Geometry check sheet. Reference: the model listing, model coordinates, mm. A direction names the side the tool comes from. Coordinates: 2 decimals unless noted, no trailing zeros. Loops run counter-clockwise (first coordinate to the right, second up) from the corner with the lowest first, then second, coordinate; pieces in that order, holes last. Notation, with made-up numbers: (13.25, -20.75) -> (35.25, -20.75) arc R24 ccw to (35.25, 8.25) -> close; hole circle Ø1 at (-14.5, 89). An arc over 180 degrees is marked (long way). Answer as a JSON object with one key per item and string values.
from build123d import *

# Parameters (mm, degrees)
F0_R     = 48.035646
F1_DEPTH = 18


with BuildPart() as f1:
    # F0 (on Front) → F1 (new body)
    with BuildSketch(Plane.XZ):
        Polygon((-1152.091861, -39.495662), (52.929014, -39.495662), (52.929014, 361.01982), (-1152.091861, 1360.379338), align=None)
        with Locations((-1022.033925, 72.34408)):
            Circle(F0_R, mode=Mode.SUBTRACT)
        with Locations((-862.033925, 72.34408)):
            Circle(F0_R, mode=Mode.SUBTRACT)
        with Locations((-1022.033925, 232.34408)):
            Circle(F0_R, mode=Mode.SUBTRACT)
        with Locations((-862.033925, 232.34408)):
            Circle(F0_R, mode=Mode.SUBTRACT)
        with Locations((-702.033925, 72.34408)):
            Circle(F0_R, mode=Mode.SUBTRACT)
        with Locations((-702.033925, 232.34408)):
            Circle(F0_R, mode=Mode.SUBTRACT)
        with Locations((-1022.033925, 392.34408)):
            Circle(F0_R, mode=Mode.SUBTRACT)
        with Locations((-862.033925, 392.34408)):
            Circle(F0_R, mode=Mode.SUBTRACT)
        with Locations((-1022.033925, 552.34408)):
            Circle(F0_R, mode=Mode.SUBTRACT)
        with Locations((-862.033925, 552.34408)):
            Circle(F0_R, mode=Mode.SUBTRACT)
        with Locations((-702.033925, 392.34408)):
            Circle(F0_R, mode=Mode.SUBTRACT)
        with Locations((-702.033925, 552.34408)):
            Circle(F0_R, mode=Mode.SUBTRACT)
        with Locations((-542.033925, 72.34408)):
            Circle(F0_R, mode=Mode.SUBTRACT)
        with Locations((-382.033925, 72.34408)):
            Circle(F0_R, mode=Mode.SUBTRACT)
        with Locations((-542.033925, 232.34408)):
            Circle(F0_R, mode=Mode.SUBTRACT)
        with Locations((-382.033925, 232.34408)):
            Circle(F0_R, mode=Mode.SUBTRACT)
        with Locations((-222.033925, 72.34408)):
            Circle(F0_R, mode=Mode.SUBTRACT)
        with Locations((-62.033925, 72.34408)):
            Circle(F0_R, mode=Mode.SUBTRACT)
        with Locations((-222.033925, 232.34408)):
            Circle(F0_R, mode=Mode.SUBTRACT)
        with Locations((-62.033925, 232.34408)):
            Circle(F0_R, mode=Mode.SUBTRACT)
        with Locations((-542.033925, 392.34408)):
            Circle(F0_R, mode=Mode.SUBTRACT)
        with Locations((-382.033925, 392.34408)):
            Circle(F0_R, mode=Mode.SUBTRACT)
        with Locations((-542.033925, 552.34408)):
            Circle(F0_R, mode=Mode.SUBTRACT)
        with Locations((-382.033925, 552.34408)):
            Circle(F0_R, mode=Mode.SUBTRACT)
        with Locations((-222.033925, 392.34408)):
            Circle(F0_R, mode=Mode.SUBTRACT)
        with Locations((-1022.033925, 712.34408)):
            Circle(F0_R, mode=Mode.SUBTRACT)
        with Locations((-862.033925, 712.34408)):
            Circle(F0_R, mode=Mode.SUBTRACT)
        with Locations((-702.033925, 712.34408)):
            Circle(F0_R, mode=Mode.SUBTRACT)
        Polygon((-588.994136, 827.545822), (-1101.989508, 827.545822), (-1101.989508, 1252.988085), align=None, mode=Mode.SUBTRACT)
        with Locations((-542.033925, 712.34408)):
            Circle(F0_R, mode=Mode.SUBTRACT)
    extrude(amount=F1_DEPTH)


solid = f1.part
1. Thickness scan on probe 1 along Z at (x, y) = (-537.5, -4.25); probe 2 along Z at (x, y) = (-539, -11.5); probe 3 along Z at (x, y) = (-341, -13.5). Record the ranges inside material, lowest first. Write a range as from..to.
Evaluation:
{"probe 1": "z = -39.5..24.52, 120.17..184.52, 280.17..344.52, 440.17..504.52, 600.17..664.52, 760.17..850.68", "probe 2": "z = -39.5..24.4, 120.28..184.4, 280.28..344.4, 440.28..504.4, 600.28..664.4, 760.28..851.92", "probe 3": "z = -39.5..47.37, 97.32..207.37, 257.32..367.37, 417.32..527.37, 577.32..687.72"}
2. Section check C-C, the plane y = -3. State how many separate pieces and enclosed holes the cut face has, then the cut area to 3 significant figures.
Evaluation:
{"separate pieces": "1", "enclosed holes": "30", "area": "765,000 mm^2"}
3. Tool access check on faces 1 (the face through (-849.083, -8.874, 1043.245)), 2 (the face through (-826, 0, 515)). Record the directions out of +Z, -Z, +X, -X, +Y, -Y that give a thin tool (end or side, any length) a straight path to the whole face; none if there is none.
Evaluation:
{"face 1": "+Y, -Y", "face 2": "+Z, -Z, +X, -X, +Y"}
4. Depth check by flat-ended pin: P1, Ø3, axis at x = -576, y = -4.5, coming from the +Z side; P2, Ø1, axis at y = -12.5, z = 704, coming from the +X side. Enter the tip coordinate at first touch or a pass-through.
Evaluation:
{"P1": "stops at z = 883.85", "P2": "stops at x = -360.03"}
5. Section check B-B, the plane z = 912.5. Record the boundary of the cut face in (x, y).
Evaluation:
{"outline": "(-1152.09, -18) -> (-1101.99, -18) -> (-1101.99, 0) -> (-1152.09, 0) -> close; (-691.43, -18) -> (-612.04, -18) -> (-612.04, 0) -> (-691.43, 0) -> close"}
6. Section check A-A, the plane x = -870. Record the boundary of the cut face in (y, z).
Evaluation:
{"outline": "(-18, -39.5) -> (0, -39.5) -> (0, 24.97) -> (-18, 24.97) -> close; (-18, 119.71) -> (0, 119.71) -> (0, 184.97) -> (-18, 184.97) -> close; (-18, 279.71) -> (0, 279.71) -> (0, 344.97) -> (-18, 344.97) -> close; (-18, 439.71) -> (0, 439.71) -> (0, 504.97) -> (-18, 504.97) -> close; (-18, 599.71) -> (0, 599.71) -> (0, 664.97) -> (-18, 664.97) -> close; (-18, 759.71) -> (0, 759.71) -> (0, 827.55) -> (-18, 827.55) -> close; (-18, 1060.59) -> (0, 1060.59) -> (0, 1126.43) -> (-18, 1126.43) -> close"}
7. Mould release check, pull along X, two halves, no side actions. Record for faces 3 (the face through (-1070.023, -8.874, 74.456)), 4 (the face through (-541.146, -8.874, 853.704)), 5 (the face through (-826, -18, 515)): released by +X, released by -X, zero draft, split by the parting line, or undercut.
Evaluation:
{"face 3": "undercut", "face 4": "released by +X", "face 5": "zero draft"}
